```python
from build123d import *

# Parameters (mm, degrees)
F0_W     = 136
F0_H     = 82
F1_DEPTH = 12
F2_W     = 48
F2_H     = 82
F3_DEPTH = 4
F4_W     = 48
F4_H     = 82
F5_DEPTH = 4
F6_R     = 14
F7_R     = 5.5
F8_DEPTH = 16.001
F9_R     = 3


with BuildPart() as f1:
    # F0 (on Front) → F1 (new body)
    with BuildSketch(Plane.XZ):
        with Locations((68, 41)):
            Rectangle(F0_W, F0_H)
    extrude(amount=F1_DEPTH)

    # F2 (on face) → F3 (join)
    with BuildSketch(Plane.XZ.offset(12)):
        with Locations((68, 41)):
            Rectangle(F2_W, F2_H)
    extrude(amount=F3_DEPTH)

    # F4 (on face) → F5 (cut)
    with BuildSketch(Plane(origin=(0, 0, 0), x_dir=(-1, 0, 0), z_dir=(0, 1, 0))):
        with Locations((-68.19709, 41)):
            Rectangle(F4_W, F4_H)
    extrude(amount=-F5_DEPTH, mode=Mode.SUBTRACT)

    # F6
    f6_edges = [f1.edges().sort_by_distance(p)[0] for p in [
        (136, -6, 82),
        (0, -6, 82),
        (136, -6, 0),
        (0, -6, 0),
    ]]
    fillet(f6_edges, radius=F6_R)

    # F7 (on Front) → F8 (cut, through all)
    with BuildSketch(Plane.XZ):
        with BuildLine():
            Line((121.913074, 62.5), (121.913074, 73.5))
            ThreePointArc((121.913074, 73.5), (116.413074, 68), (121.913074, 62.5))
        make_face()
        with BuildLine():
            ThreePointArc((127.413074, 68), (125.802162, 71.889087), (121.913074, 73.5))
            Line((121.913074, 73.5), (121.913074, 62.5))
            ThreePointArc((121.913074, 62.5), (125.802162, 64.110913), (127.413074, 68))
        make_face()
        with BuildLine():
            ThreePointArc((127.413074, 14), (125.802162, 17.889087), (121.913074, 19.5))
            Line((121.913074, 19.5), (121.913074, 8.5))
            ThreePointArc((121.913074, 8.5), (125.802162, 10.110913), (127.413074, 14))
        make_face()
        with BuildLine():
            Line((121.913074, 8.5), (121.913074, 19.5))
            ThreePointArc((121.913074, 19.5), (116.413074, 14), (121.913074, 8.5))
        make_face()
        with Locations((13.913074, 14)):
            Circle(F7_R)
        with Locations((13.913074, 68)):
            Circle(F7_R)
    extrude(amount=F8_DEPTH, mode=Mode.SUBTRACT)

    # F9
    f9_edges = [f1.edges().sort_by_distance(p)[0] for p in [
        (92.19709, -4, 41),
        (44.19709, -4, 41),
    ]]
    fillet(f9_edges, radius=F9_R)


solid = f1.part
```
Can you work these out from the model? Positions are in its coordinate system, mm. A direction names the side the tool comes from. Round coordinates to 2 decimals unless told otherwise and drop trailing zeros. Loops run counter-clockwise (first coordinate to the right, second up) from the corner with the lowest first, then second, coordinate; pieces in that order, holes last. Notation, with made-up numbers: M 73,-21.75 L 120,-21.75 A21 cw 120,-9.75 Z; hole C 19,77 d2. An arc over 180 degrees is marked long. Write item = value, one per line. Start each with the question number.
(1) I'm going to push flat-ended pins straight in: P1, Ø1, axis at x = 17.5, z = 18.5, coming from the -Y side; P2, Ø1.2, axis at y = -14, z = 38.5, coming from the +X side; P3, Ø4, axis at x = 55, z = 65.5, coming from the +Y side. Where does each tip first touch, or does it pass through?
(2) If we mould it in two halves opening along X, with no side actions, what happens to faces 4 (the face through (131.8, -6.1, 4)), 5 (the face through (67, -8, 82)), 6 (the face through (45.053, -3.098, 41.574))? For each: released by +X, released by -X, zero draft, split by the parting line, or undercut.
(3) Which directions (+Z, -Z, +X, -X, +Y, -Y) give clear straight access to the entire face, cutting with the end or side of a thin tool? Please do faces 1 (the face through (22, -12, 42)), 2 (the face through (114, -12, 42)), 3 (the face through (68, -4, 42)).
(4) I need wall thicknesses on line 1 along X through (y, z) = (-10, 14); line 2 along X through (y, z) = (-1.25, 60.5); line 3 along Z through (x, y) = (17.5, -7). Which ranges of each line are inside material? Lowest first, please.
(5) Suppose I cut it at B-B on z = 59. Write out the boundary of the cut face in (x, y).
(6) Suppose I cut it at A-A on y = -9. Write out the boundary of the cut face in (x, z).
(7) Suppose I cut it at C-C on x = 120. Write out the boundary of the cut face in (y, z), plus the area to 3 significant figures.
(8) Suppose I cut it at D-D on z = 18. Write out the boundary of the cut face in (x, y), plus the area to 3 significant figures.
Answer block:
q1.P1 = -12
q1.P2 = 92
q1.P3 = -4
q2.face_4 = released by +X
q2.face_5 = zero draft
q2.face_6 = undercut
q3.face_1 = +Z, -Z, -X, -Y
q3.face_2 = +Z, -Z, +X, -Y
q3.face_3 = +Z, -Z, +Y
q4.line_1 = 0 to 8.41, 19.41 to 116.41, 127.41 to 136
q4.line_2 = 0 to 44.21, 92.19 to 136
q4.line_3 = 0 to 9.83, 18.17 to 63.83, 72.17 to 82
q5.outline = M 0,-12 L 44,-12 L 44,-16 L 92,-16 L 92,-12 L 136,-12 L 136,0 L 92.2,0 L 92.2,-1 A3 cw 89.2,-4 L 47.2,-4 A3 cw 44.2,-1 L 44.2,0 L 0,0 Z
q6.outline = M 0,14 A14 ccw 14,0 L 122,0 A14 ccw 136,14 L 136,68 A14 ccw 122,82 L 14,82 A14 ccw 0,68 Z; hole C 13.91,14 d11; hole C 13.91,68 d11; hole M 121.91,8.5 A5.5 ccw 127.41,14 A5.5 ccw long Z; hole M 121.91,62.5 A5.5 ccw 127.41,68 A5.5 ccw long Z
q7.outline = M -12,0 L 0,0 L 0,8.84 L -12,8.84 Z; M -12,19.16 L 0,19.16 L 0,62.84 L -12,62.84 Z; M -12,73.16 L 0,73.16 L 0,82 L -12,82 Z
q7.area = 736 mm²
q8.outline = M 0,-12 L 10.14,-12 L 10.14,0 L 0,0 Z; M 17.69,-12 L 44,-12 L 44,-16 L 92,-16 L 92,-12 L 118.14,-12 L 118.14,0 L 92.2,0 L 92.2,-1 A3 cw 89.2,-4 L 47.2,-4 A3 cw 44.2,-1 L 44.2,0 L 17.69,0 Z; M 125.69,-12 L 136,-12 L 136,0 L 125.69,0 Z
q8.area = 1,450 mm²
